Here's how the part is built. I have some questions about the finished solid (model axes, mm). Coordinates: 2 decimals unless noted, no trailing zeros. Write each loop counter-clockwise with the first axis right and the second up, starting at its lowest first coordinate (ties: lowest second). Pieces come first, ordered by that corner, then holes. Notation, with made-up numbers: (30.5, 22.5) -> (82.5, 22.5) arc R25 cw to (82.5, 56.5) -> close; hole circle Ø11 at (-29.5, 43.25). An arc over 180 degrees is marked (long way). Put each result on its own line as item: value.
Autodesk Inventor part; units mm, degrees
ref_plane "YZ Plane" through (0, 0, 0) normal (1, 0, 0) x (0, 1, 0)
ref_plane "XZ Plane" through (0, 0, 0) normal (0, 1, 0) x (-1, 0, 0)
ref_plane "XY Plane" through (0, 0, 0) normal (0, 0, 1) x (1, 0, 0)
sketch "スケッチ1" plane through (0, 0, 0) normal (0, 0, 1) x (1, 0, 0)
  line L0 (-2, 0.75) -> (-2, 3)
  line L1 (2, 3) -> (2, 0.75)
  line L2 (-2, 0.75) -> (2, 0.75)
  line L3 (-2, 3) -> (-1, 3)
  line L4 (2, 3) -> (1, 3)
  line L5 (-1, 3) -> (-1, 2.5)
  line L6 (1, 3) -> (1, 2.5)
  arc A0 (-1, 2.5) -> (1, 2.5) centre (0, 2.5) ccw
  line L7 (0, 2.5) -> (0, 0.75) construction
  line L8 (-2.8, 0) -> (2.8, 0)
  point P0 (0, 0)
  dimension "d0" = 0.75
  dimension "d3" = 1
  dimension "d4" = 0.5
  dimension "d5" = 3
  dimension "d7" = 1
revolve "回転1" add sketch "スケッチ1" angle 360 about axis through (-10, 0, 0) along (1, 0, 0)
properties part number "Pulley_Small"
Item 1: Imagine slicing it at A-A on z = 0. Write out the boundary of the cut face in (x, y).
Output:
outline: (-2, -3) -> (-1, -3) -> (-1, -2.5) arc R1 cw to (1, -2.5) -> (1, -3) -> (2, -3) -> (2, -0.75) -> (-2, -0.75) -> close; (-2, 0.75) -> (2, 0.75) -> (2, 3) -> (1, 3) -> (1, 2.5) arc R1 cw to (-1, 2.5) -> (-1, 3) -> (-2, 3) -> close
Item 2: Imagine slicing it at D-D on x = 1.75. Write out the boundary of the cut face in (y, z).
Output:
outline: circle Ø6 at (0, 0); hole circle Ø1.5 at (0, 0)
Item 3: Imagine slicing it at C-C on x = -0.8. Write out the boundary of the cut face in (y, z), then the cut area to 3 significant figures.
Output:
outline: circle Ø3.8 at (0, 0); hole circle Ø1.5 at (0, 0)
area: 9.57 mm²
Item 4: If we mould it in two halves opening along X, with no side actions, what happens to faces 1 (the flat face through (-1, -2, 2)), 2 (the flat face through (1, -2, 2)), 3 (the cylindrical face through (-1.5, -3, 0.1)), 4 (the flat face through (-2, 1, -1))? For each: released by +X, released by -X, zero draft, split by the parting line, or undercut.
Output:
face 1: undercut
face 2: undercut
face 3: zero draft
face 4: released by -X
Item 5: Please list where these lines run through material, in increasing order: line 1 along Z through (x, y) = (1.15, 0); line 2 along X through (y, z) = (-0.4, -2.6); line 3 along X through (y, z) = (1.55, -0.9). Write a range as from..to.
Output:
line 1: z = -3..-0.75, 0.75..3
line 2: x = -2..-1, 1..2
line 3: x = -2..-0.71, 0.71..2
